```python
from build123d import *

# Parameters (mm, degrees)
SKETCH1_R           = 3.525
BOSS_EXTRUDE1_DEPTH = 6


with BuildPart() as part:
    # Sketch1 → Boss-Extrude1 (new body)
    with BuildSketch(Plane(origin=(0, 0, 0), x_dir=(1, 0, 0), z_dir=(0, 1, 0))):
        with BuildLine():
            Line((-56.916994756, 70.5), (-24.883005244, 70.5))
            ThreePointArc((-24.883005244, 70.5), (-14.3, 78.5), (-3.716994756, 70.5))
            Line((-3.716994756, 70.5), (1.716994756, 70.5))
            ThreePointArc((1.716994756, 70.5), (12.3, 78.5), (22.883005244, 70.5))
            Line((22.883005244, 70.5), (56.916994756, 70.5))
            ThreePointArc((56.916994756, 70.5), (75.278174593, 75.278174593), (70.5, 56.916994756))
            Line((70.5, 56.916994756), (70.5, 44.833005244))
            ThreePointArc((70.5, 44.833005244), (78.5, 34.25), (70.5, 23.666994756))
            Line((70.5, 23.666994756), (70.5, -15.016994756))
            ThreePointArc((70.5, -15.016994756), (78.5, -25.6), (70.5, -36.183005244))
            Line((70.5, -36.183005244), (70.5, -56.916994756))
            ThreePointArc((70.5, -56.916994756), (75.278174593, -75.278174593), (56.916994756, -70.5))
            Line((56.916994756, -70.5), (36.183005244, -70.5))
            ThreePointArc((36.183005244, -70.5), (25.6, -78.5), (15.016994756, -70.5))
            Line((15.016994756, -70.5), (-23.666994756, -70.5))
            ThreePointArc((-23.666994756, -70.5), (-34.25, -78.5), (-44.833005244, -70.5))
            Line((-44.833005244, -70.5), (-56.916994756, -70.5))
            ThreePointArc((-56.916994756, -70.5), (-75.278174593, -75.278174593), (-70.5, -56.916994756))
            Line((-70.5, -56.916994756), (-70.5, -22.883005244))
            ThreePointArc((-70.5, -22.883005244), (-78.5, -12.3), (-70.5, -1.716994756))
            Line((-70.5, -1.716994756), (-70.5, 3.716994756))
            ThreePointArc((-70.5, 3.716994756), (-78.5, 14.3), (-70.5, 24.883005244))
            Line((-70.5, 24.883005244), (-70.5, 56.916994756))
            ThreePointArc((-70.5, 56.916994756), (-75.278174593, 75.278174593), (-56.916994756, 70.5))
        make_face()
        with Locations(Location((-32.5, 32.5, 0), (0, 0, 270))):
            Circle(SKETCH1_R, mode=Mode.SUBTRACT)
        with Locations(Location((32.5, 32.5, 0), (0, 0, 270))):
            Circle(SKETCH1_R, mode=Mode.SUBTRACT)
        with Locations(Location((32.5, -32.5, 0), (0, 0, 270))):
            Circle(SKETCH1_R, mode=Mode.SUBTRACT)
        with Locations(Location((-32.5, -32.5, 0), (0, 0, 270))):
            Circle(SKETCH1_R, mode=Mode.SUBTRACT)
        with BuildLine():
            Line((36.183005244, -64.5), (56.916994756, -64.5))
            ThreePointArc((56.916994756, -64.5), (59.721825407, -59.721825407), (64.5, -56.916994756))
            Line((64.5, -56.916994756), (64.5, -36.183005244))
            ThreePointArc((64.5, -36.183005244), (60.514437119, -34.097170779), (57.697103802, -30.590313229))
            Line((57.697103802, -30.590313229), (40.909272567, -33.899914244))
            ThreePointArc((40.909272567, -33.899914244), (38.52808531, -38.52808531), (33.899914244, -40.909272567))
            Line((33.899914244, -40.909272567), (30.590313229, -57.697103802))
            ThreePointArc((30.590313229, -57.697103802), (34.097170779, -60.514437119), (36.183005244, -64.5))
        make_face(mode=Mode.SUBTRACT)
        with BuildLine():
            Line((-56.916994756, 64.5), (-24.883005244, 64.5))
            ThreePointArc((-24.883005244, 64.5), (-23.702757073, 61.791396017), (-21.844148835, 59.49463815))
            Line((-21.844148835, 59.49463815), (-31.480193598, 40.963782836))
            ThreePointArc((-31.480193598, 40.963782836), (-38.52808531, 38.52808531), (-40.963782836, 31.480193598))
            Line((-40.963782836, 31.480193598), (-59.49463815, 21.844148835))
            ThreePointArc((-59.49463815, 21.844148835), (-61.791396017, 23.702757073), (-64.5, 24.883005244))
            Line((-64.5, 24.883005244), (-64.5, 56.916994756))
            ThreePointArc((-64.5, 56.916994756), (-59.721825407, 59.721825407), (-56.916994756, 64.5))
        make_face(mode=Mode.SUBTRACT)
        with BuildLine():
            Line((-64.5, -56.916994756), (-64.5, -22.883005244))
            ThreePointArc((-64.5, -22.883005244), (-61.999259001, -21.825851587), (-59.833621297, -20.188386247))
            Line((-59.833621297, -20.188386247), (-40.910840036, -31.10953429))
            ThreePointArc((-40.910840036, -31.10953429), (-39.986708997, -36.577353724), (-35.894744259, -40.319931996))
            Line((-35.894744259, -40.319931996), (-36.717766955, -56.780385909))
            ThreePointArc((-36.717766955, -56.780385909), (-41.831475725, -59.529979559), (-44.833005244, -64.5))
            Line((-44.833005244, -64.5), (-56.916994756, -64.5))
            ThreePointArc((-56.916994756, -64.5), (-59.721825407, -59.721825407), (-64.5, -56.916994756))
        make_face(mode=Mode.SUBTRACT)
        with BuildLine():
            Line((-3.716994756, 64.5), (1.716994756, 64.5))
            ThreePointArc((1.716994756, 64.5), (6.799259001, 57.974148413), (14.991767169, 56.834429715))
            Line((14.991767169, 56.834429715), (25.912915211, 37.911648453))
            ThreePointArc((25.912915211, 37.911648453), (28.422646276, 25.013291003), (40.619557697, 29.902230226))
            Line((40.619557697, 29.902230226), (57.080011611, 30.725252921))
            ThreePointArc((57.080011611, 30.725252921), (59.918524275, 26.279979559), (64.5, 23.666994756))
            Line((64.5, 23.666994756), (64.5, -15.016994756))
            ThreePointArc((64.5, -15.016994756), (59.002829221, -18.614437119), (56.536583679, -24.703616953))
            Line((56.536583679, -24.703616953), (39.748752444, -28.013217968))
            ThreePointArc((39.748752444, -28.013217968), (26.47191469, -26.47191469), (28.013217968, -39.748752444))
            Line((28.013217968, -39.748752444), (24.703616953, -56.536583679))
            ThreePointArc((24.703616953, -56.536583679), (18.614437119, -59.002829221), (15.016994756, -64.5))
            Line((15.016994756, -64.5), (-23.666994756, -64.5))
            ThreePointArc((-23.666994756, -64.5), (-26.279979559, -59.918524275), (-30.725252921, -57.080011611))
            Line((-30.725252921, -57.080011611), (-29.902230226, -40.619557697))
            ThreePointArc((-29.902230226, -40.619557697), (-25.013291003, -28.422646276), (-37.911648453, -25.912915211))
            Line((-37.911648453, -25.912915211), (-56.834429715, -14.991767169))
            ThreePointArc((-56.834429715, -14.991767169), (-57.974148413, -6.799259001), (-64.5, -1.716994756))
            Line((-64.5, -1.716994756), (-64.5, 3.716994756))
            ThreePointArc((-64.5, 3.716994756), (-58.097242927, 8.591396017), (-56.72652173, 16.520848028))
            Line((-56.72652173, 16.520848028), (-38.195666417, 26.156892791))
            ThreePointArc((-38.195666417, 26.156892791), (-26.47191469, 26.47191469), (-26.156892791, 38.195666417))
            Line((-26.156892791, 38.195666417), (-16.520848028, 56.72652173))
            ThreePointArc((-16.520848028, 56.72652173), (-8.591396017, 58.097242927), (-3.716994756, 64.5))
        make_face(mode=Mode.SUBTRACT)
        with BuildLine():
            Line((22.883005244, 64.5), (56.916994756, 64.5))
            ThreePointArc((56.916994756, 64.5), (59.721825407, 59.721825407), (64.5, 56.916994756))
            Line((64.5, 56.916994756), (64.5, 44.833005244))
            ThreePointArc((64.5, 44.833005244), (59.529979559, 41.831475725), (56.780385909, 36.717766955))
            Line((56.780385909, 36.717766955), (40.319931996, 35.894744259))
            ThreePointArc((40.319931996, 35.894744259), (36.577353724, 39.986708997), (31.10953429, 40.910840036))
            Line((31.10953429, 40.910840036), (20.188386247, 59.833621297))
            ThreePointArc((20.188386247, 59.833621297), (21.825851587, 61.999259001), (22.883005244, 64.5))
        make_face(mode=Mode.SUBTRACT)
    extrude(amount=BOSS_EXTRUDE1_DEPTH)


solid = part.part
```
Source: CAD feature listing. Evaluate the final solid. Frame: model axes, mm. A direction names the side the tool comes from. Give positions to 0.01 mm unless a question says otherwise; leave off trailing zeros. Loops run counter-clockwise (first coordinate to the right, second up) from the corner with the lowest first, then second, coordinate; pieces in that order, holes last. Notation, with made-up numbers: (-26, 8.25) -> (-6, 8.25) arc R36 cw to (-6, 46.25) -> close; hole circle Ø6 at (18, 66.25). An arc over 180 degrees is marked (long way). Use a Markdown table: item, result. Add a question column.
(1) Access query for faces 4 (the face through (32.268, 2.958, 49.186)), 5 (the face through (-78.5, 3, 12.5)). Directions: +Z, -Z, +X, -X, +Y, -Y. A direction counts if a zero-diameter tool reaches every point of the face in a straight line with its end or side. Return the directions, or none.
(2) Section query D-D (x = -51). Output: boundary loops of the cut face in (y, z), then the cut area to 3 significant figures.
(3) First-contact query: pin 1 Ø3 at (y, z) = (4.5, 39) entering from -X; pin 2 Ø1.8 at (x, y) = (-52.5, 4) entering from -Z; pin 3 Ø1.8 at (y, z) = (2, -10) entering from -X; pin 4 Ø6.5 at (x, z) = (32.5, 32.5) entering from -Y. Flat tips, straight axial feed; report the tip coordinate or a pass-through.
(4) Section query B-B (z = 60.5). Output: boundary loops of the cut face in (x, y), then the cut area to 3 significant figures.
(5) Pull-direction query (X, two-part tool) for faces 1 (the face through (-70.5, 3, -41)), 2 (the face through (-57.915, 2.958, 6.902)), 3 (the face through (-58.16, 2.96, -8.49)); classes: +X half, -X half, draft (parallel to the pull), parting line (faces both ways), or undercut.
(6) Ray query, line 1 (Z direction, x = -0.5, y = 1.2); line 2 (X direction, y = 5.1, z = -35); line 3 (Z direction, x = -71.5, y = 5.3). Return the intervals inside material, ascending.
(7) Section query A-A (x = -18.5). Output: boundary loops of the cut face in (y, z).
(8) Section query C-C (y = 1.45). Count the separate pieces of the cut face and the enclosed holes in it, then the cut area to 3 significant figures.
Checked values:
| question | item | result |
|---|---|---|
| 1 | face 4 | +Y, -Y |
| 1 | face 5 | -X, +Y, -Y |
| 2 | outline | (0, -70.5) -> (6, -70.5) -> (6, -64.5) -> (0, -64.5) -> close; (0, -26.26) -> (6, -26.26) -> (6, -19.5) -> (0, -19.5) -> close; (0, 18.36) -> (6, 18.36) -> (6, 25.29) -> (0, 25.29) -> close; (0, 64.5) -> (6, 64.5) -> (6, 70.5) -> (0, 70.5) -> close |
| 2 | area | 154 mm^2 |
| 3 | pin 1 | x = -70.5 |
| 3 | pin 2 | z = -70.5 |
| 3 | pin 3 | x = -77.96 |
| 3 | pin 4 | through |
| 4 | outline | (-75.99, 0) -> (-59.01, 0) -> (-59.01, 6) -> (-75.99, 6) -> close; (-42.74, 0) -> (-25.76, 0) -> (-25.76, 6) -> (-42.74, 6) -> close; (17.11, 0) -> (34.09, 0) -> (34.09, 6) -> (17.11, 6) -> close; (59.01, 0) -> (75.99, 0) -> (75.99, 6) -> (59.01, 6) -> close |
| 4 | area | 407 mm^2 |
| 5 | face 1 | -X half |
| 5 | face 2 | undercut |
| 5 | face 3 | undercut |
| 6 | line 1 | -70.5 to -64.5, 64.5 to 70.5 |
| 6 | line 2 | -70.5 to -64.5, -40.65 to -34.99, -30.01 to -24.35, 24.35 to 30.01, 34.99 to 78.47 |
| 6 | line 3 | -77.75 to -57.25, -24.55 to -4.05, 2.05 to 22.55, 57.25 to 77.75 |
| 7 | outline | (0, -77.67) -> (6, -77.67) -> (6, -52.92) -> (0, -52.92) -> close; (0, 64.5) -> (6, 64.5) -> (6, 70.5) -> (0, 70.5) -> close |
| 8 | separate pieces | 1 |
| 8 | enclosed holes | 9 |
| 8 | area | 7,880 mm^2 |
